Drawing for the job (mm, zero at the part's lowest x, y, z). A direction names the side the tool comes from. Give positions to 0.01 mm unless a question says otherwise; leave off trailing zeros. Loops run counter-clockwise (first coordinate to the right, second up) from the corner with the lowest first, then second, coordinate; pieces in that order, holes last. Notation, with made-up numbers: (-23, 2.25) -> (2, 2.25) arc R23 ccw to (2, 37.25) -> close; hole circle Ø11 at (48.5, 38). An arc over 180 degrees is marked (long way). Write item = value, one per line.
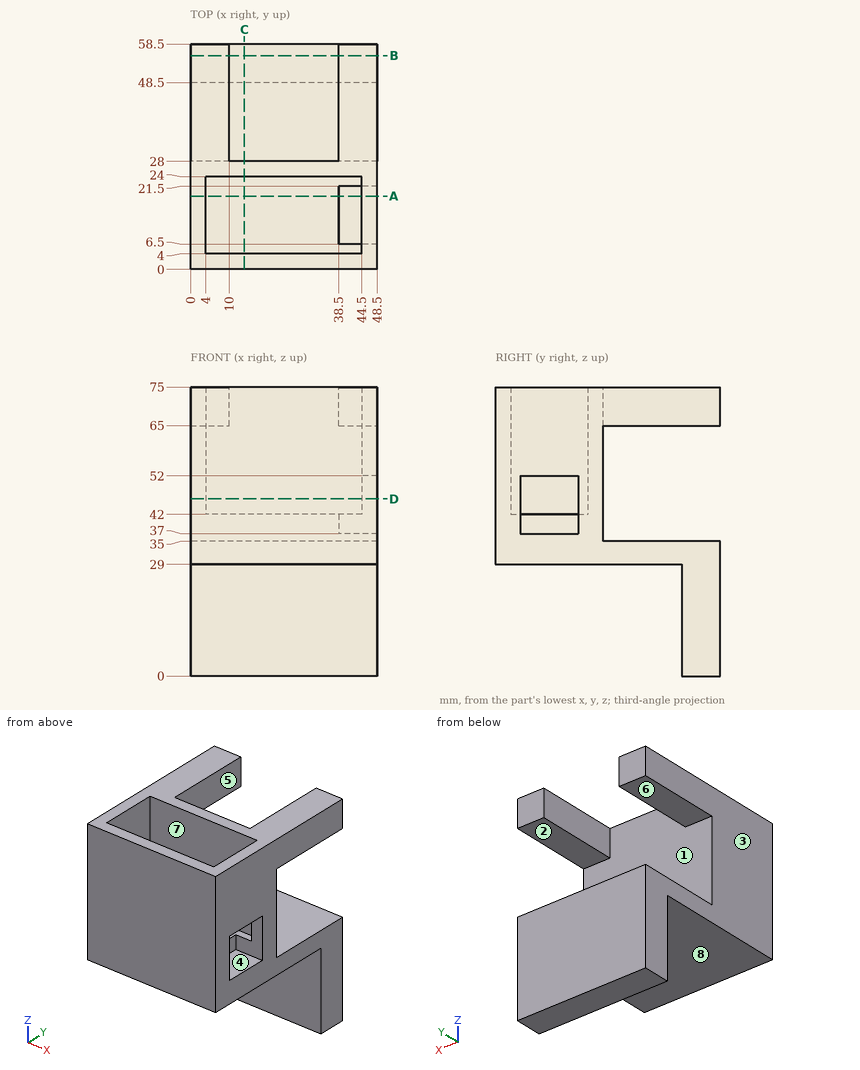
1) Pull direction X, two halves, no side cores. Call the marked faces 1, 2 and 3: pulls with the +X half, pulls with the -X half, needs draft (parallel to the pull), parting line crosses it, or undercut.
Resolved:
face_1 = undercut
face_2 = needs draft
face_3 = pulls with the -X half
2) Which spindle directions (+Z, -Z, +X, -X, +Y, -Y) get a long thin tool onto all of the face, cutting with end or side? Do the marked faces 4, 5, 6, 7 and 8. Say none if no direction does.
Resolved:
face_4 = +X
face_5 = +Z, +Y
face_6 = +X, -X, +Y
face_7 = +Z
face_8 = -Z, +X, -X, -Y
3) Slice it at C-C, the plane x = 14. List the corners of the cut face in (y, z).
Resolved:
outline = (0, 29) -> (48.5, 29) -> (48.5, 0) -> (58.5, 0) -> (58.5, 35) -> (28, 35) -> (28, 75) -> (24, 75) -> (24, 42) -> (4, 42) -> (4, 75) -> (0, 75) -> close
4) Slice it at D-D, the plane z = 46. List the corners of the cut face in (x, y), and give its area (3 significant figures).
Resolved:
outline = (0, 0) -> (48.5, 0) -> (48.5, 6.5) -> (44.5, 6.5) -> (44.5, 4) -> (4, 4) -> (4, 24) -> (44.5, 24) -> (44.5, 21.5) -> (48.5, 21.5) -> (48.5, 28) -> (0, 28) -> close
area = 488 mm²
5) Slice it at B-B, the plane y = 55.5. List the corners of the cut face in (x, z).
Resolved:
outline = (0, 0) -> (48.5, 0) -> (48.5, 35) -> (0, 35) -> close; (0, 65) -> (10, 65) -> (10, 75) -> (0, 75) -> close; (38.5, 65) -> (48.5, 65) -> (48.5, 75) -> (38.5, 75) -> close
6) Drill centre lines: line 1 along X through (y, z) = (13, 58.5); line 2 along Y through (x, z) = (35.5, 60.5); line 3 along Z through (x, y) = (6.5, 46). Where is each one in solid material? Low to high. Write a range as [from, to].
Resolved:
line_1 = [0, 4], [44.5, 48.5]
line_2 = [0, 4], [24, 28]
line_3 = [29, 35], [65, 75]
7) Drop flat-ended pins along their axis: P1, Ø24, axis at x = 32, y = 20.5, coming from the -Z side; P2, Ø9, axis at x = 28, y = 45, coming from the +Z side; P3, Ø6, axis at x = 25.5, y = 17, coming from the +Z side. Give the stop position or say it passes through.
Resolved:
P1 = 29
P2 = 35
P3 = 42
8) Slice it at A-A, the plane y = 19. List the corners of the cut face in (x, z).
Resolved:
outline = (0, 29) -> (48.5, 29) -> (48.5, 37) -> (38.5, 37) -> (38.5, 42) -> (4, 42) -> (4, 75) -> (0, 75) -> close; (44.5, 52) -> (48.5, 52) -> (48.5, 75) -> (44.5, 75) -> close
